```python
from build123d import *

# Parameters (mm, degrees)
F1_DEPTH  = 500
F2_W      = 2
F2_H      = 21
F3_DEPTH  = 20
F4_R      = 2.5
F5_DEPTH  = 25
F6_R      = 10
F7_R      = 2.5
F8_DEPTH  = 25
F9_R      = 2.5
F10_DEPTH = 25


with BuildPart() as f1:
    # F0 (on Top) → F1 (new body)
    with BuildSketch(Plane.XY):
        Polygon((-46.834455, -41.400001), (-46.834455, -43.400001), (-21.834455, -43.400001), (-21.834455, -18.400001), (-46.834455, -18.400001), (-46.834455, -20.400001), (-23.834455, -20.400001), (-23.834455, -41.400001), align=None)
    extrude(amount=F1_DEPTH)

    # F2 (on face) → F3 (cut)
    with BuildSketch(Plane(origin=(0, 0, 0), x_dir=(1, 0, 0), z_dir=(0, 0, -1))):
        with Locations((-22.834455, 30.900001)):
            Rectangle(F2_W, F2_H)
    extrude(amount=-F3_DEPTH, mode=Mode.SUBTRACT)

    # F4 (on face) → F5 (cut)
    with BuildSketch(Plane.XZ.offset(43.400001)):
        with Locations((-31.834455, 10)):
            Circle(F4_R)
    extrude(amount=-F5_DEPTH, mode=Mode.SUBTRACT)

    # F6
    f6_edges = [f1.edges().sort_by_distance(p)[0] for p in [
        (-46.834455, -19.400001, 0),
        (-46.834455, -42.400001, 0),
        (-46.834455, -42.400001, 500),
        (-46.834455, -19.400001, 500),
        (-21.834455, -42.400001, 0),
        (-21.834455, -19.400001, 0),
    ]]
    fillet(f6_edges, radius=F6_R)

    # F7 (on face) → F8 (cut)
    with BuildSketch(Plane.YZ.offset(-21.834455)):
        with Locations((-30.900001, 490)):
            Circle(F7_R)
    extrude(amount=-F8_DEPTH, mode=Mode.SUBTRACT)

    # F9 (on face) → F10 (cut)
    with BuildSketch(Plane.XZ.offset(43.400001)):
        with Locations((-34.334455, 60)):
            Circle(F9_R)
    extrude(amount=-F10_DEPTH, mode=Mode.SUBTRACT)


solid = f1.part
```
Geometry check sheet. Reference: the model listing, model coordinates, mm. A direction names the side the tool comes from. Coordinates: 2 decimals unless noted, no trailing zeros. Order: outer loops, then holes, each group sorted by start corner. A loop starts at its lowest first (then second) coordinate and runs counter-clockwise, first axis right, second up.
Item 1: Section check A-A (z = 428). Enter the section's corners in (x, y), plus the area to 3 significant figures.
Item 2: Tool access check on faces 4 (the cylindrical face through (-43.983, -42.414, 3.007)), 5 (the flat face through (-23.834, -31, 257)). Record the directions out of +Z, -Z, +X, -X, +Y, -Y that give a thin tool (end or side, any length) a straight path to the whole face; none if there is none.
Item 3: Scan lines: line 1 along Y through (x, z) = (-32.75, 300); line 2 along Y through (x, z) = (-22.9, 490); line 3 along X through (y, z) = (-33.25, 215). Record each from-to range of solid material in increasing order.
Item 4: Depth check by flat-ended pin: pin 1 (1 mm diameter, centred on y = -37.5, z = 308, fed in from -X); pin 2 (1 mm diameter, centred on x = -23, y = -28, fed in from -Z). Enter the tip coordinate at first touch or a pass-through.
Item 5: Mould release check, pull along Y, two halves, no side actions. Record for faces 1 (the flat face through (-37, -41.4, 246)), 2 (the flat face through (-35, -43.4, 246)), 3 (the cylindrical face through (-43.983, -42.414, 496.993)): released by +Y, released by -Y, zero draft, split by the parting line, or undercut.
Item 6: Section check B-B (x = -41). Enter the section's corners in (y, z), plus the area to 3 significant figures.
Check sheet entries:
1. outline: (-46.83, -43.4) - (-21.83, -43.4) - (-21.83, -18.4) - (-46.83, -18.4) - (-46.83, -20.4) - (-23.83, -20.4) - (-23.83, -41.4) - (-46.83, -41.4) - close
1. area: 142 mm2
2. face 4: -Z, -X, +Y, -Y
2. face 5: +Z, -Z, -X
3. line 1: y = -43.4 to -41.4, -20.4 to -18.4
3. line 2: y = -43.4 to -33.4, -28.4 to -18.4
3. line 3: x = -23.83 to -21.83
4. pin 1: stops at x = -23.83
4. pin 2: stops at z = 20
5. face 1: undercut
5. face 2: released by -Y
5. face 3: zero draft
6. outline: (-43.4, 0.91) - (-41.4, 0.91) - (-41.4, 499.09) - (-43.4, 499.09) - close; (-20.4, 0.91) - (-18.4, 0.91) - (-18.4, 499.09) - (-20.4, 499.09) - close
6. area: 1,990 mm2
